```python
from build123d import *

# Parameters (mm, degrees)
F0_R      = 0.9
F1_DEPTH  = 3
F5_W      = 1.6
F5_H      = 8
F6_DEPTH  = 9
F7_R      = 0.9
F8_DEPTH  = 11.2
F9_R      = 2.4
F10_DEPTH = 15
F11_R     = 1.5


with BuildPart() as f1:
    # F0 (on Top) → F1 (new body)
    with BuildSketch(Plane.XY):
        with BuildLine():
            Line((-1.414214, 11.313708), (-6.363961, 6.363961))
            ThreePointArc((-6.363961, 6.363961), (0, -9), (6.363961, 6.363961))
            Line((6.363961, 6.363961), (1.414214, 11.313708))
            ThreePointArc((1.414214, 11.313708), (0, 11.899495), (-1.414214, 11.313708))
        make_face()
        with Locations((0, 9.899495)):
            Circle(F0_R, mode=Mode.SUBTRACT)
    extrude(amount=F1_DEPTH)

    # F2 (on Right) → F3 (revolve)
    with BuildSketch(Plane.YZ):
        with BuildLine():
            Line((0, 10), (0, 3))
            Line((0, 3), (9, 3))
            ThreePointArc((9, 3), (7.163441, 7.497235), (3, 10))
            Line((3, 10), (0, 10))
        make_face()
        with BuildLine():
            Line((9, 0), (0, 0))
            Line((0, 0), (0, -80))
            Line((0, -80), (1, -80))
            ThreePointArc((1, -80), (1.707107, -79.707107), (2, -79))
            Line((2, -79), (2, -40))
            Line((2, -40), (9, 0))
        make_face()
    revolve(axis=Axis((0, 0, -40), (0, 0, -1)))

    # F5 (on offset) → F6 (cut)
    with BuildSketch(Plane.XZ.offset(-9)):
        with Locations((0, -72.8)):
            Rectangle(F5_W, F5_H)
    extrude(amount=F6_DEPTH, mode=Mode.SUBTRACT)

    # F7 (on face) → F8 (cut)
    with BuildSketch(Plane(origin=(0, 0, -80), x_dir=(1, 0, 0), z_dir=(0, 0, -1))):
        Circle(F7_R)
    extrude(amount=-F8_DEPTH, mode=Mode.SUBTRACT)

    # F9 (on face) → F10 (join)
    with BuildSketch(Plane.XY.offset(10)):
        Circle(F9_R)
    extrude(amount=F10_DEPTH)

    # F11
    f11_edges = [f1.edges().sort_by_distance(p)[0] for p in [
        (-2.4, 0, 25),
    ]]
    fillet(f11_edges, radius=F11_R)


solid = f1.part
```
Here's how the part is built. I have some questions about the finished solid (model axes, mm). A direction names the side the tool comes from. Give positions to 0.01 mm unless a question says otherwise; leave off trailing zeros. Loops run counter-clockwise (first coordinate to the right, second up) from the corner with the lowest first, then second, coordinate; pieces in that order, holes last. Notation, with made-up numbers: M -31,88.25 L 11,88.25 A15 ccw 11,108.25 Z; hole C 64.25,59.25 d1. An arc over 180 degrees is marked long. Use one line per item in the form item = value. Start each with the question number.
Q1. I need wall thicknesses on line 1 along X through (y, z) = (0, -76); line 2 along Z through (x, y) = (-2, 10.5); line 3 along Y through (x, z) = (-3.5, -11). Which ranges of each line are inside material? Lowest first, please.
Q2. Will these pins go through, and if not, where does the flat tip stop? pin 1 Ø1 at (y, z) = (-3.5, -44.5) entering from -X; pin 2 Ø1.5 at (x, z) = (-6.5, -9.5) entering from +Y; pin 3 Ø6 at (x, y) = (-1, 9) entering from +Z; pin 4 Ø8 at (x, z) = (4, -31.5) entering from -Y.
Q3. Which directions (+Z, -Z, +X, -X, +Y, -Y) give clear straight access to the entire face, cutting with the end or side of a thin tool? Please do faces 4 (the cylindrical face through (0, -2, -59)), 5 (the cylindrical face through (0, -9, 1)), 6 (the flat face through (0, 0, 25)), 7 (the flat face through (-1, 9.3, 0)), 8 (the cylindrical face through (1.29, 2.024, 16.656)).
Q4. If we section it at B-B (z = -55): Write out the boundary of the cut face in (x, y).
Q5. If we section it at A-A (z = -38): Write out the boundary of the cut face in (x, y), then the cut area to 3 significant figures.
Q6. Thinking about a two-plate mould opening in Y: for faces 1 (the flat face through (-1, 9.3, 3)), 2 (the flat face through (-3.854, 8.873, 1.479)), 3 (the cylindrical face through (-0.12, 10.79, 1.48)), which applies, +Y half, -Y half, draft (parallel to the pull), parting line (faces both ways), or undercut?
Taken from the geometry:
q1.line_1 = -2 to -0.9, 0.9 to 2
q1.line_2 = 0 to 3
q1.line_3 = -6.15 to 6.15
q2.pin_1 = through
q2.pin_2 = 4.58
q2.pin_3 = 8.56
q2.pin_4 = -3.83
q3.face_4 = -Z
q3.face_5 = +Z, -Z
q3.face_6 = +Z, +X, -X, +Y, -Y
q3.face_7 = -Z, +Y
q3.face_8 = +Z
q4.outline = C 0,0 d4
q5.outline = C 0,0 d4.7
q5.area = 17.3 mm^2
q6.face_1 = draft
q6.face_2 = +Y half
q6.face_3 = undercut
